from build123d import *

# Parameters (mm, degrees)
BOSS_EXTRUDE1_DEPTH      = 30
SKETCH2_R                = 9
BOSS_EXTRUDE2_DEPTH      = 12
BOSS_EXTRUDE2_DEPTH_BACK = 24
FILLET1_R                = 5
BOSS_EXTRUDE3_DEPTH      = 12
RIB1_REACH               = 80
SKETCH4_WALL_W           = 230.993150364
SKETCH4_WALL_H           = 12
CUT_EXTRUDE1_DEPTH       = 25


with BuildPart() as part:
    # Sketch1 → Boss-Extrude1 (new body, symmetric)
    with BuildSketch(Plane.XY):
        Polygon((0, 0), (0, 24), (72, 24), (72, 13), (49, 13), (49, 0), (37, 0), (37, 13), (12, 13), (12, 0), align=None)
    extrude(amount=BOSS_EXTRUDE1_DEPTH, both=True)

    # Sketch2 → Boss-Extrude2 (add, two sides)
    with BuildSketch(Plane(origin=(0, 24, 0), x_dir=(1, 0, 0), z_dir=(0, 1, 0))) as boss_extrude2_sk:
        with BuildLine():
            Line((72, 30), (72, -30))
            ThreePointArc((72, -30), (104.696938457, -40.392304845), (84, -13.029437252))
            Line((84, -13.029437252), (84, 13.029437252))
            ThreePointArc((84, 13.029437252), (104.696938457, 40.392304845), (72, 30))
        make_face()
        with Locations(Location((90, 30, 0), (0, 0, 270))):  # turned: the seam where the file's is
            Circle(SKETCH2_R, mode=Mode.SUBTRACT)
        with Locations(Location((90, -30, 0), (0, 0, 270))):  # turned: the seam where the file's is
            Circle(SKETCH2_R, mode=Mode.SUBTRACT)
    extrude(amount=BOSS_EXTRUDE2_DEPTH)
    extrude(boss_extrude2_sk.sketch, amount=-BOSS_EXTRUDE2_DEPTH_BACK)

    # Fillet1
    fillet1_edges = [part.edges().sort_by_distance(p)[0] for p in [
        (84, 18, -13.029437252),
        (84, 18, 13.029437252),
    ]]
    fillet(fillet1_edges, radius=FILLET1_R)

    # Sketch3 → Boss-Extrude3 (add)
    with BuildSketch(Plane.XZ):
        with BuildLine():
            Line((108, 30), (108, -30))
            ThreePointArc((108, -30), (102.448153347, -16.998327867), (89.217391304, -12.01702128))
            ThreePointArc((89.217391304, -12.01702128), (85.542179626, -10.633325006), (84, -7.021749414))
            Line((84, -7.021749414), (84, 7.021749414))
            ThreePointArc((84, 7.021749414), (85.542179626, 10.633325006), (89.217391304, 12.01702128))
            ThreePointArc((89.217391304, 12.01702128), (102.448153347, 16.998327867), (108, 30))
        make_face()
    extrude(amount=-BOSS_EXTRUDE3_DEPTH)

    # Sketch4 wall → Rib1 (add, up to next)
    with BuildSketch(Plane(origin=(36, 30, -30), x_dir=(-0.986393924, -0.164398987, 0), z_dir=(-0.164398987, 0.986393924, 0)), mode=Mode.PRIVATE) as rib1_sk1:
        with Locations((0, 6)):
            Rectangle(SKETCH4_WALL_W, SKETCH4_WALL_H)
    rib1_tool1 = extrude(rib1_sk1.sketch, amount=-RIB1_REACH, mode=Mode.PRIVATE) - part.part
    add(rib1_tool1.solids().sort_by_distance((36, 30, -30))[0])

    # Sketch5 → Cut-Extrude1 (cut, through all)
    with BuildSketch(Plane(origin=(0, 24, 0), x_dir=(1, 0, 0), z_dir=(0, 1, 0))):
        with BuildLine():
            Line((33, 1), (33, -8))
            ThreePointArc((33, -8), (25, -16), (17, -8))
            Line((17, -8), (17, 1))
            ThreePointArc((17, 1), (25, 9), (33, 1))
        make_face()
    extrude(amount=-CUT_EXTRUDE1_DEPTH, mode=Mode.SUBTRACT)


solid = part.part
Geometry check sheet. Reference: the model listing, model coordinates, mm. A direction names the side the tool comes from. Round coordinates to 2 decimals unless told otherwise and drop trailing zeros. Write each loop counter-clockwise with the first axis right and the second up, starting at its lowest first coordinate (ties: lowest second). Pieces come first, ordered by that corner, then holes. Notation, with made-up numbers: (27.5, -19.75) - (79.5, -19.75) arc R37 cw to (79.5, 18.25) - close; hole circle Ø9 at (24.5, 30). An arc over 180 degrees is marked (long way). One line per item, written item: value.
1. Cross-section at B-B on x = 15. Record the boundary of the cut face in (y, z).
The answers:
outline: (13, -30) - (26.5, -30) - (26.5, -18) - (24, -18) - (24, 30) - (13, 30) - close
2. Cross-section at A-A on y = 3.5. Record the boundary of the cut face in (x, z), and give its area (3 significant figures).
The answers:
outline: (0, -30) - (12, -30) - (12, 30) - (0, 30) - close; (37, -30) - (49, -30) - (49, 30) - (37, 30) - close; (72, -30) arc R18 ccw to (108, -30) - (108, 30) arc R18 ccw to (72, 30) - close; hole circle Ø18 at (90, -30); hole circle Ø18 at (90, 30)
area: 4,110 mm^2
3. Cross-section at D-D on y = 28.5. Record the boundary of the cut face in (x, z).
The answers:
outline: (27, -30) - (72, -30) arc R18 ccw (long way) to (89.22, -12.02) arc R5 cw to (84, -7.02) - (84, 7.02) arc R5 cw to (89.22, 12.02) arc R18 ccw (long way) to (72, 30) - (72, -18) - (27, -18) - close; hole circle Ø18 at (90, -30); hole circle Ø18 at (90, 30)
4. Scan lines: L1, parallel to X at y = 24.5, z = 29.5; L2, parallel to X at y = 11.5, z = 26; L3, parallel to Z at x = 46.5, y = 6.5. Record each from-to range of solid material in increasing order.
The answers:
L1: x = 72 to 81.01, 98.99 to 107.99
L2: x = 0 to 12, 37 to 49, 72 to 81.94, 98.06 to 108
L3: z = -30 to 30
5. Cross-section at C-C on z = -26. Record the boundary of the cut face in (x, y), and give its area (3 significant figures).
The answers:
outline: (0, 0) - (12, 0) - (12, 13) - (37, 13) - (37, 0) - (49, 0) - (49, 13) - (72, 13) - (72, 0) - (81.94, 0) - (81.94, 36) - (72, 36) - (0, 24) - close; (98.06, 0) - (108, 0) - (108, 12) - (107.55, 12) - (107.55, 36) - (98.06, 36) - close
area: 2,240 mm^2
6. Set-up check for faces 1 (the face through (16, 13, 0)), 2 (the face through (99, 12, 0)), 3 (the face through (25, 19, 16)), 4 (the face through (95.53, 18.25, -47.13)), 5 (the face through (45, 27, -18)): record each of +Z, -Z, +X, -X, +Y, -Y from which the full face is reachable in a straight line by a thin tool's end or side.
The answers:
face 1: +Z, -Z, -Y
face 2: +X, +Y
face 3: +Y, -Y
face 4: +Y
face 5: +Z, -X, +Y
7. Mould release check, pull along Z, two halves, no side actions. Record for faces 6 (the face through (82, 36, -1)), 7 (the face through (85.5, 24.17, 10.59)), 8 (the face through (37, 18, -30)): released by +Z, released by -Z, zero draft, split by the parting line, or undercut.
The answers:
face 6: zero draft
face 7: undercut
face 8: released by -Z
8. Depth check by flat-ended pin: pin 1 Ø4 at (x, z) = (30, -21) entering from +Y; pin 2 Ø12.5 at (x, z) = (19.5, 11.5) entering from -Y; pin 3 Ø7 at (x, y) = (39.5, 8.5) entering from +Z. Enter the tip coordinate at first touch or a pass-through.
The answers:
pin 1: stops at y = 29.33
pin 2: stops at y = 13
pin 3: stops at z = 30
